Design review of the part built by this model. Coordinates are the model's own, in mm. Coordinates: 2 decimals unless noted, no trailing zeros. Loops run counter-clockwise (first coordinate to the right, second up) from the corner with the lowest first, then second, coordinate; pieces in that order, holes last.
Autodesk Inventor part; units mm, degrees
ref_plane "YZ Plane" through (0, 0, 0) normal (1, 0, 0) x (0, 1, 0)
ref_plane "XZ Plane" through (0, 0, 0) normal (0, 1, 0) x (-1, 0, 0)
ref_plane "XY Plane" through (0, 0, 0) normal (0, 0, 1) x (1, 0, 0)
sketch "Skizze1" plane through (0, 0, 0) normal (0, 0, 1) x (1, 0, 0)
  line L0 (-16.1655, 0) -> (16.1655, 0)
  line L1 (0, -14.0455) -> (0, 14.0455)
  line L2 (-5.7168, 10.0325) -> (5.83, 9.9672)
  line L3 (5.83, 9.9672) -> (11.5468, -0.0653)
  line L4 (11.5468, -0.0653) -> (5.7168, -10.0325)
  line L5 (5.7168, -10.0325) -> (-5.83, -9.9672)
  line L6 (-5.83, -9.9672) -> (-11.5468, 0.0653)
  line L7 (-11.5468, 0.0653) -> (-5.7168, 10.0325)
  point P0 (0, 0)
  point P1 (0, 0)
  dimension "d0" = 20
extrude "Extrusion1" add sketch "Skizze1" along normal blind 50
sketch "Skizze2" plane through (-5.7168, 10.0325, 50) normal (0.0056567, 0.999984, 0) x (0.999984, -0.0056567, 0)
  line L0 (11.547, 0) -> (0, 0)
  circle A0 centre (5.7735, 25) radius 2.5
  point P0 (5.7735, 50)
  dimension "d3" = 25
  dimension "d4" = 5
extrude "Extrusion2" cut sketch "Skizze2" against normal blind 10
sketch "Skizze3" plane through (0, 0, 0) normal (0, 0, -1) x (-1, 0, 0)
  point P0 (0, 0)
hole "Bohrung1" at (0, 0, 0) direction (0, 0, 1) diameter 11.445 depth 40
sketch "Skizze4" plane through (0, 0, 50) normal (0, 0, 1) x (1, 0, 0)
  point P0 (0, 0)
hole "Bohrung2" at (0, 0, 50) direction (0, 0, -1) diameter 11.445 depth 40
chamfer "Fase1" distance 0.5 angle 45 1 edges at (0, -5.7225, 0)
chamfer "Fase2" distance 0.5 angle 45 1 edges at (0, 5.7225, 50)
sketch "Skizze5" plane through (0, 0, 50) normal (0, 0, 1) x (1, 0, 0)
  point P0 (0, 0)
properties part number "Luftregler1"
Q1. Clearance check with flat-ended pins moving along their axes: pin 1 Ø9 at (x, y) = (0, 0) entering from +Z; pin 2 Ø1.5 at (x, z) = (4.5, 19.5) entering from +Y; pin 3 Ø8 at (x, z) = (-6, 34.5) entering from -Y; pin 4 Ø3 at (y, z) = (2.5, 42) entering from -X. State where each tip first meets the part, or that it passes through.
Q2. The part is to be moulded in two halves that separate along Z. For faces 1 (the cylindrical face through (-2.454, 7.622, 24.89)), 2 (the flat face through (8.65, 5.02, 24.65)), 3 (the flat face through (5, -4, 50)), say which applies: pulls with the +Z half, pulls with the -Z half, needs draft (parallel to the pull), parting line crosses it, or undercut.
Q3. Take a section at A-A, the plane z = 32.5. Write out the cut boundary in (x, y) (1 decimal).
Q4. For line 1 (X direction, y = 3.75, z = 41); line 2 (X direction, y = 0, z = 4); line 3 (Y direction, x = 0, z = 8), list the stretches that pass through material, from the lowest coordinate up.
Q5. Take a section at D-D, the plane y = -7.5. Write out the cut boundary in (x, z), then the cut area to 3 significant figures.
Q6. Take a section at C-C, the plane x = -9. Write out the cut boundary in (y, z), then the cut area to 3 significant figures.
Q7. Take a section at B-B, the plane x = -0.5. Give the number of separate pieces and of enclosed holes in the cut face, then the cut area to 3 significant figures.
Entries:
1. pin 1: passes through
1. pin 2: stops at y = 9.98
1. pin 3: stops at y = -9.99
1. pin 4: stops at x = -11
2. face 1: undercut
2. face 2: needs draft
2. face 3: pulls with the +Z half
3. outline: (-11.5, 0.1) - (-5.8, -10) - (5.7, -10) - (11.5, -0.1) - (5.8, 10) - (-5.7, 10) - close; hole circle Ø11.4 at (0, 0)
4. line 1: x = -9.39 to -4.32, 4.32 to 9.37
4. line 2: x = -11.51 to -5.72, 5.72 to 11.51
4. line 3: y = -10 to -5.72, 5.72 to 10
5. outline: (-7.24, 0) - (7.2, 0) - (7.2, 50) - (-7.24, 50) - close
5. area: 722 mm2
6. outline: (-4.4, 0) - (4.42, 0) - (4.42, 50) - (-4.4, 50) - close
6. area: 441 mm2
7. separate pieces: 3
7. enclosed holes: 0
7. area: 408 mm2
